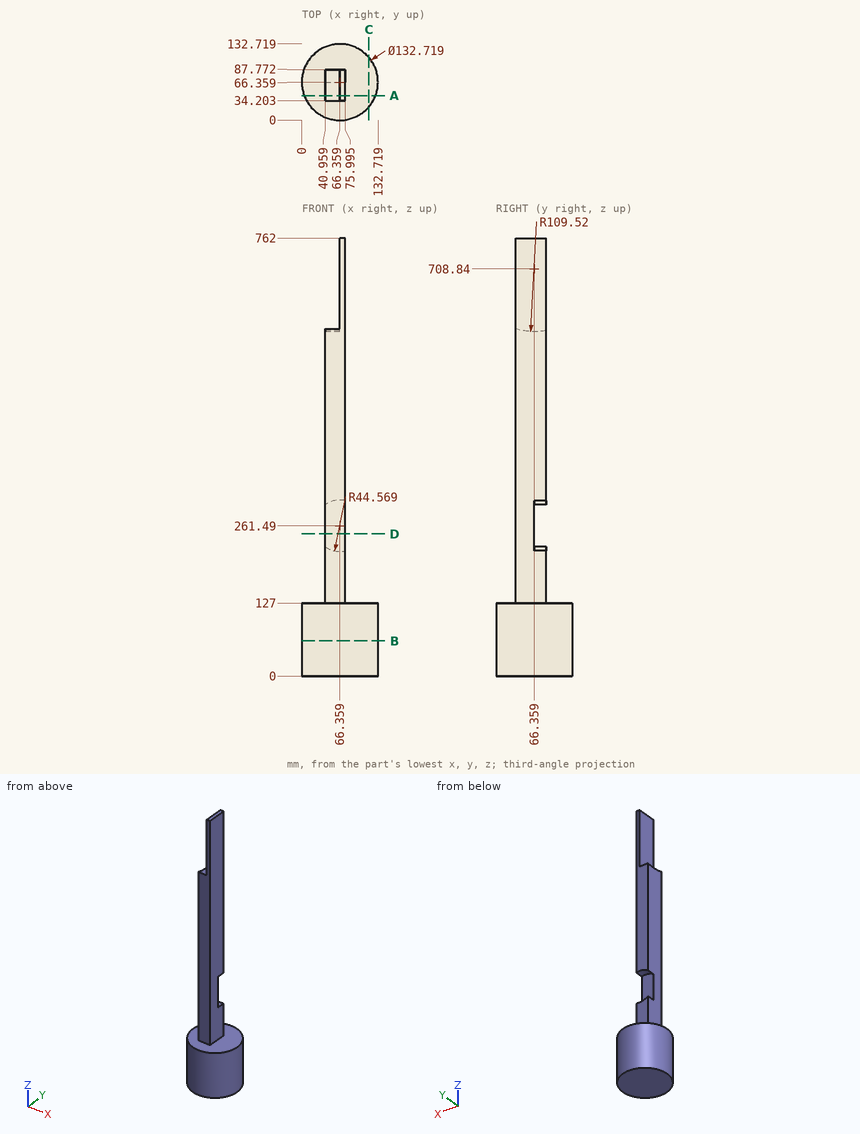
Geometry check sheet. Reference: drawing and pictorial views, mm from the part's lowest x, y, z. Coordinates: 2 decimals unless noted, no trailing zeros. Write each loop counter-clockwise with the first axis right and the second up, starting at its lowest first coordinate (ties: lowest second). Pieces come first, ordered by that corner, then holes. Notation, with made-up numbers: (41.25, -21) -> (72.25, -21) arc R18 cw to (72.25, 12) -> close; hole circle Ø5 at (7, 28). An arc over 180 degrees is marked (long way). Use a Markdown table: item, result.
1. Sectioned sample at D-D (z = 247.5). Enter the section's corners in (x, y) (1 decimal), plus the area to 3 significant figures.
Reported:
| item | result |
|---|---|
| outline | (41, 34.2) -> (76, 34.2) -> (76, 66.4) -> (41, 66.4) -> close |
| area | 1,130 mm2 |
2. Scan lines: line 1 along X through (y, z) = (68, 657.5) (1 decimal); line 2 along Y through (x, z) = (65, 68) (1 decimal); line 3 along Z through (x, y) = (126, 91). Record each from-to range of solid material in increasing order.
Reported:
| item | result |
|---|---|
| line 1 | x = 66.4 to 76 |
| line 2 | y = 0 to 132.7 |
| line 3 | z = 0 to 127 |
3. Sectioned sample at A-A (y = 43). Enter the section's corners in (x, z) (1 decimal), plus the area to 3 significant figures.
Reported:
| item | result |
|---|---|
| outline | (4.2, 0) -> (128.5, 0) -> (128.5, 127) -> (76, 127) -> (76, 762) -> (66.4, 762) -> (66.4, 601.8) -> (41, 601.8) -> (41, 127) -> (4.2, 127) -> close |
| area | 34,000 mm2 |
4. Sectioned sample at C-C (x = 117). Enter the section's corners in (y, z) (1 decimal).
Reported:
| item | result |
|---|---|
| outline | (23.5, 0) -> (109.2, 0) -> (109.2, 127) -> (23.5, 127) -> close |
5. Go/stop test with flat-tipped pins: pin 1 Ø2 at (y, z) = (41, 87.5) entering from -X; pin 2 Ø12 at (x, z) = (40.5, 300) entering from +Y; pin 3 Ø12 at (x, z) = (46.5, 316.5) entering from -Y; pin 4 Ø1.5 at (x, y) = (51.5, 18) entering from -Z. Record where each tip stops, or that it passes through.
Reported:
| item | result |
|---|---|
| pin 1 | stops at x = 4.63 |
| pin 2 | stops at y = 87.77 |
| pin 3 | stops at y = 34.2 |
| pin 4 | stops at z = 0 |
6. Sectioned sample at B-B (z = 61). Enter the section's corners in (x, y), plus the area to 3 significant figures.
Reported:
| item | result |
|---|---|
| outline | circle Ø132.72 at (66.36, 66.36) |
| area | 13,800 mm2 |
